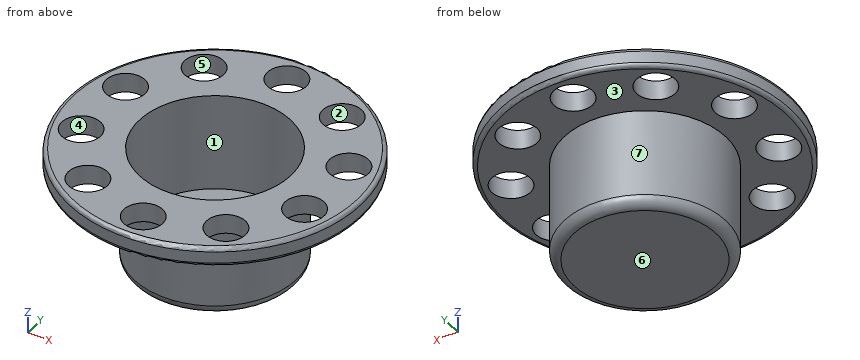
```python
from build123d import *

# Parameters (mm, degrees)
SKETCH2_R           = 75
SKETCH2_R_2         = 40
EXTRUDE_THIN1_DEPTH = 10
SKETCH3_R           = 41.655
SKETCH3_R_2         = 39.005
EXTRUDE_THIN2_DEPTH = 60
SKETCH4_R           = 39.005
BOSS_EXTRUDE1_DEPTH = 10
SKETCH5_R           = 10
CUT_EXTRUDE1_DEPTH  = 11
FILLET1_R           = 5
FILLET2_R           = 2


with BuildPart() as part:
    # Sketch2 → Extrude-Thin1 (new body)
    with BuildSketch(Plane.XY):
        Circle(SKETCH2_R)
        Circle(SKETCH2_R_2, mode=Mode.SUBTRACT)
    extrude(amount=EXTRUDE_THIN1_DEPTH)

    # Sketch3 → Extrude-Thin2 (add)
    with BuildSketch(Plane.XY.offset(10)):
        Circle(SKETCH3_R)
        Circle(SKETCH3_R_2, mode=Mode.SUBTRACT)
    extrude(amount=-EXTRUDE_THIN2_DEPTH)

    # Sketch4 → Boss-Extrude1 (add)
    with BuildSketch(Plane(origin=(0, 0, -50), x_dir=(-1, 0, 0), z_dir=(0, 0, -1))):
        Circle(SKETCH4_R)
    extrude(amount=-BOSS_EXTRUDE1_DEPTH)

    # Sketch5 → Cut-Extrude1 (cut, through all)
    with BuildSketch(Plane(origin=(0, 0, 0), x_dir=(-1, 0, 0), z_dir=(0, 0, -1))):
        with Locations((0, 60)):
            Circle(SKETCH5_R)
        with Locations((35.267115138, 48.541019662)):
            Circle(SKETCH5_R)
        with Locations((57.063390978, 18.541019662)):
            Circle(SKETCH5_R)
        with Locations((57.063390978, -18.541019662)):
            Circle(SKETCH5_R)
        with Locations((35.267115138, -48.541019662)):
            Circle(SKETCH5_R)
        with Locations((0, -60)):
            Circle(SKETCH5_R)
        with Locations((-35.267115138, -48.541019662)):
            Circle(SKETCH5_R)
        with Locations((-57.063390978, -18.541019662)):
            Circle(SKETCH5_R)
        with Locations((-57.063390978, 18.541019662)):
            Circle(SKETCH5_R)
        with Locations((-35.267115138, 48.541019662)):
            Circle(SKETCH5_R)
    extrude(amount=-CUT_EXTRUDE1_DEPTH, mode=Mode.SUBTRACT)

    # Fillet1
    fillet1_edges = [part.edges().sort_by_distance(p)[0] for p in [
        (-41.655, 0, -50),
    ]]
    fillet(fillet1_edges, radius=FILLET1_R)

    # Fillet2
    fillet2_edges = [part.edges().sort_by_distance(p)[0] for p in [
        (-75, 0, 0),
        (-75, 0, 10),
    ]]
    fillet(fillet2_edges, radius=FILLET2_R)


solid = part.part
```
Read the model definition and answer for the solid it produces. Units are mm, in the model's axes. Face numbers are marked on the shaded views. A direction names the side the tool comes from. Coordinates: 2 decimals unless noted, no trailing zeros. Loops run counter-clockwise (first coordinate to the right, second up) from the corner with the lowest first, then second, coordinate; pieces in that order, holes last.
(1) A tool of negligible diameter and unlimited length cuts with its end or side. For the marked faces 1, 2 and 3, from which of +Z, -Z, +X, -X, +Y, -Y can it reach the whole face along a straight path? Write none if from no direction.
Solution:
face 1: +Z
face 2: +Z, -Z
face 3: -Z
(2) The part is cut by section C-C (x = -0.5). Count the separate pieces of the cut face and the enclosed holes in it, and give its area (3 significant figures).
Solution:
separate pieces: 3
enclosed holes: 0
area: 1,350 mm2
(3) The part is cut by section B-B (z = -9). Determine the outline of the cut face in (x, y) (3 decimals), and give its area (3 significant figures).
Solution:
outline: circle Ø83.31 at (0, 0); hole circle Ø78.01 at (0, 0)
area: 672 mm2
(4) Consider line 1 along Y through (x, z) = (0, 7.5) (3 decimals); line 2 along X through (y, z) = (43.5, 6.5); line 3 along Z through (x, y) = (-12, -28.5). Determine where each line is inside the solid, lowest interval first.
Solution:
line 1: y = -75 to -70, -50 to -39.005, 39.005 to 50, 70 to 75
line 2: x = -61.1 to -43.9, -26.63 to 26.63, 43.9 to 61.1
line 3: z = -50 to -40
(5) The mould has two halves that part along X. Classify the marked faces 4, 5, 6 and 7: released by +X, released by -X, zero draft, split by the parting line, or undercut.
Solution:
face 4: undercut
face 5: undercut
face 6: zero draft
face 7: split by the parting line
(6) The part is cut by section A-A (y = 0). Determine the outline of the cut face in (x, z) (3 decimals).
Solution:
outline: (-75, 2) arc R2 ccw to (-73, 0) - (-41.655, 0) - (-41.655, -45) arc R5 ccw to (-36.655, -50) - (36.655, -50) arc R5 ccw to (41.655, -45) - (41.655, 0) - (73, 0) arc R2 ccw to (75, 2) - (75, 8) arc R2 ccw to (73, 10) - (39.005, 10) - (39.005, -40) - (-39.005, -40) - (-39.005, 10) - (-73, 10) arc R2 ccw to (-75, 8) - close
(7) Flat-ended cylindrical pins translate along their axes: pin 1 Ø23 at (x, y) = (-35.27, 48.54) entering from -Z; pin 2 Ø1.5 at (x, z) = (18, -0.5) entering from -Y; pin 3 Ø6 at (x, z) = (-25.5, -30) entering from -Y; pin 4 Ø23 at (x, y) = (57.06, -18.54) entering from +Z. Find the tip coordinate at first contact, or state that the pin passes through.
Solution:
pin 1: stops at z = 0
pin 2: stops at y = -71.76
pin 3: stops at y = -35.06
pin 4: stops at z = 10
